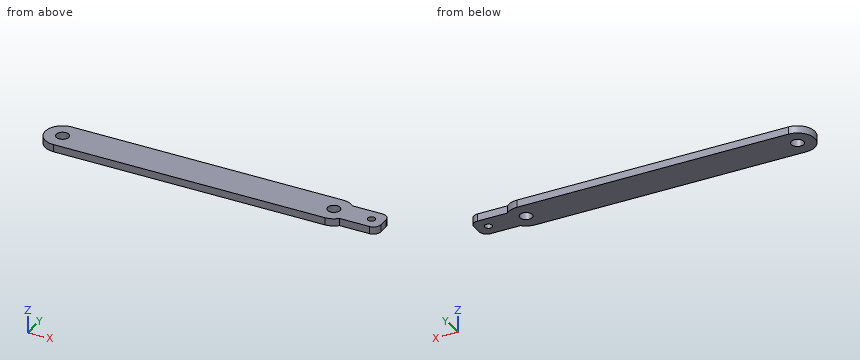
from build123d import *

# Parameters (mm, degrees)
SKETCH1_R           = 2.5
BOSS_EXTRUDE1_DEPTH = 3
SKETCH2_R           = 1.5
BOSS_EXTRUDE2_DEPTH = 3


with BuildPart() as part:
    # Sketch1 → Boss-Extrude1 (new body)
    with BuildSketch(Plane.XY):
        with BuildLine():
            Line((-70.959009299, 269.154117688), (39.040990701, 269.154117688))
            ThreePointArc((39.040990701, 269.154117688), (46.040990701, 262.154117688), (39.040990701, 255.154117688))
            Line((39.040990701, 255.154117688), (-70.959009299, 255.154117688))
            ThreePointArc((-70.959009299, 255.154117688), (-77.959009299, 262.154117688), (-70.959009299, 269.154117688))
        make_face()
        with Locations((-70.959009299, 262.154117688)):
            Circle(SKETCH1_R, mode=Mode.SUBTRACT)
        with Locations((39.040990701, 262.154117688)):
            Circle(SKETCH1_R, mode=Mode.SUBTRACT)
    extrude(amount=BOSS_EXTRUDE1_DEPTH)

    # Sketch2 → Boss-Extrude2 (add)
    with BuildSketch(Plane.XY.offset(3)):
        with BuildLine():
            Line((56.125358764, 267.154117688), (42.581100141, 267.154117688))
            Line((42.581100141, 267.154117688), (42.581100141, 257.154117688))
            Line((42.581100141, 257.154117688), (56.125358764, 257.154117688))
            ThreePointArc((56.125358764, 257.154117688), (58.246679107, 258.032797345), (59.125358764, 260.154117688))
            Line((59.125358764, 260.154117688), (59.125358764, 264.154117688))
            ThreePointArc((59.125358764, 264.154117688), (58.246679107, 266.275438032), (56.125358764, 267.154117688))
        make_face()
        with Locations((54.303681244, 262.154117688)):
            Circle(SKETCH2_R, mode=Mode.SUBTRACT)
    extrude(amount=-BOSS_EXTRUDE2_DEPTH)


solid = part.part
The listing builds one solid part. Answer for the finished solid, in the listing's coordinates (mm). Give positions to 0.01 mm unless a question says otherwise; leave off trailing zeros. Write each loop counter-clockwise with the first axis right and the second up, starting at its lowest first coordinate (ties: lowest second). Pieces come first, ordered by that corner, then holes. Notation, with made-up numbers: (51, 57) - (90, 57) arc R23 cw to (90, 91) - close; hole circle Ø3 at (-31, 38.25). An arc over 180 degrees is marked (long way). One line per question, with ' | ' between items. Start each with the question number.
1. Given P1, Ø6.5, axis at x = 39.04, y = 262.15, coming from the +Z side; P2, Ø2.5, axis at x = 54.3, y = 262.15, coming from the -Z side; P3, Ø0.9, axis at x = 53, z = 2, coming from the +Y side, each flat-ended and moving along its own axis, determine where each tip first touches the part or whether it passes through.
2. Section A-A, the plane z = 0.9 is taken. Determine the outline of the cut face in (x, y).
3. Straight lines are drawn through the part: line 1 (X direction, y = 262, z = 2.25); line 2 (X direction, y = 262.75, z = 0.7); line 3 (Y direction, x = -69.5, z = 1.65). For each, find the intervals that lie inside material, in ascending order.
4. Section B-B, the plane x = 47 is taken. Determine the outline of the cut face in (y, z).
Result:
1) P1: stops at z = 3 | P2: passes through | P3: stops at y = 267.15
2) outline: (-70.96, 255.15) - (39.04, 255.15) arc R7 ccw to (43.94, 257.15) - (56.13, 257.15) arc R3 ccw to (59.13, 260.15) - (59.13, 264.15) arc R3 ccw to (56.13, 267.15) - (43.94, 267.15) arc R7 ccw to (39.04, 269.15) - (-70.96, 269.15) arc R7 ccw to start; hole circle Ø5 at (-70.96, 262.15); hole circle Ø5 at (39.04, 262.15); hole circle Ø3 at (54.3, 262.15)
3) line 1: x = -77.96 to -73.45, -68.46 to 36.55, 41.54 to 52.81, 55.8 to 59.13 | line 2: x = -77.93 to -73.39, -68.53 to 36.61, 41.47 to 52.93, 55.68 to 59.13 | line 3: y = 255.15 to 260.12, 264.18 to 269.15
4) outline: (257.15, 0) - (267.15, 0) - (267.15, 3) - (257.15, 3) - close
